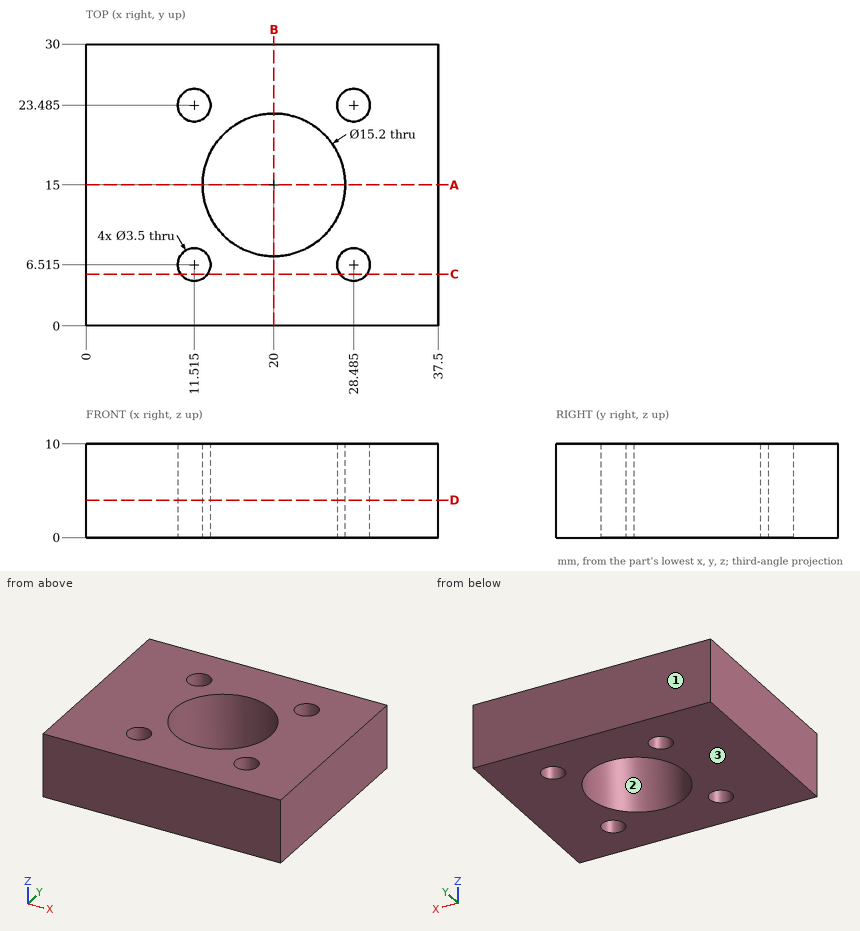
Here's the drawing with two shaded views (mm, measured from the low corner). I have some questions. Coordinates: 2 decimals unless noted, no trailing zeros. Order: outer loops, then holes, each group sorted by start corner. A loop starts at its lowest first (then second) coordinate and runs counter-clockwise, first axis right, second up. Notation, with made-up numbers: (13.5, 39) - (58.5, 39) arc R5 ccw to (58.5, 47) - close; hole circle Ø10 at (-28, -20). An arc over 180 degrees is marked (long way). Answer in a Markdown table with one row per item.
1. Suppose I cut it at B-B (x = 20). Please give me the cut outline in (y, z), and give its area (3 significant figures).
Reply:
| item | result |
|---|---|
| outline | (0, 0) - (7.4, 0) - (7.4, 10) - (0, 10) - close; (22.6, 0) - (30, 0) - (30, 10) - (22.6, 10) - close |
| area | 148 mm^2 |
2. Suppose I cut it at D-D (z = 4). Give the number of separate pieces and of enclosed holes in the cut face, and give its area (3 significant figures).
Reply:
| item | result |
|---|---|
| separate pieces | 1 |
| enclosed holes | 5 |
| area | 905 mm^2 |
3. Suppose I cut it at A-A (y = 15). Please give me the cut outline in (x, z), and give its area (3 significant figures).
Reply:
| item | result |
|---|---|
| outline | (0, 0) - (12.4, 0) - (12.4, 10) - (0, 10) - close; (27.6, 0) - (37.5, 0) - (37.5, 10) - (27.6, 10) - close |
| area | 223 mm^2 |
4. Suppose I cut it at C-C (y = 5.5). Please give me the cut outline in (x, z).
Reply:
| item | result |
|---|---|
| outline | (0, 0) - (10.09, 0) - (10.09, 10) - (0, 10) - close; (12.94, 0) - (27.06, 0) - (27.06, 10) - (12.94, 10) - close; (29.91, 0) - (37.5, 0) - (37.5, 10) - (29.91, 10) - close |
5. If we mould it in two halves opening along Y, with no side actions, what happens to the marked faces 1, 2 and 3? For each: pulls with the +Y half, pulls with the -Y half, needs draft (parallel to the pull), parting line crosses it, or undercut.
Reply:
| item | result |
|---|---|
| face 1 | pulls with the +Y half |
| face 2 | undercut |
| face 3 | needs draft |
6. If I drill on line 1 along X through (y, z) = (14.75, 3); line 2 along Y through (x, z) = (20, 2.5); line 3 along X through (y, z) = (7.25, 9.25), over which ranges is the centre line in solid material (lowest first)?
Reply:
| item | result |
|---|---|
| line 1 | x = 0 to 12.4, 27.6 to 37.5 |
| line 2 | y = 0 to 7.4, 22.6 to 30 |
| line 3 | x = 0 to 9.93, 13.1 to 26.9, 30.07 to 37.5 |
